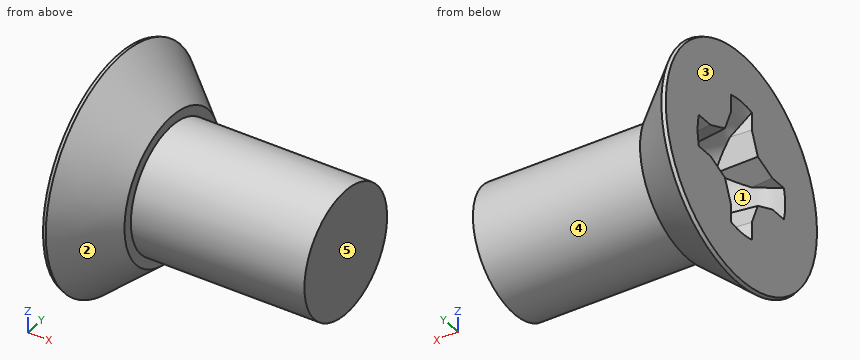
```python
from build123d import *

# Parameters (mm, degrees)
CUT_EXTRUDE1_REACH = 9.904
CIRPATTERN1_COUNT  = 4
DRAFT1_ANGLE       = 5
CHAMFER1_SIZE      = 0.133096
CHAMFER1_SIZE2     = 0.121906137


with BuildPart() as part:
    # Sketch2 → Revolve1 (revolve)
    with BuildSketch(Plane.XY, mode=Mode.PRIVATE) as revolve1_sk:
        Polygon((-3.175, 0), (3.175, 0), (3.175, 1.7526), (-1.6764, 1.7526), (-1.6764, 2.024686895), (-3.175, 3.3274), align=None)
    revolve(revolve1_sk.sketch.rotate(Axis((-3.175, 0, 0), (1, 0, 0)), 180), axis=Axis((-3.175, 0, 0), (1, 0, 0)))

    # Cut-Extrude1: up to this cone (the profile starts inside it)
    cut_extrude1_end = Plane(origin=(-3.175, 0, 0), z_dir=(-1, 0, 0)).offset(-2.137134931) * Cone(1e-06, 12.516790067, 14.398918853, align=(Align.CENTER, Align.CENTER, Align.MIN), mode=Mode.PRIVATE)
    # Sketch3 → Cut-Extrude1 (cut, up to the surface)
    with BuildSketch(Plane.ZY.offset(3.175), mode=Mode.PRIVATE) as cut_extrude1_sk1:
        with BuildLine():
            Line((0, 0), (2.218266667, 0))
            ThreePointArc((2.218266667, 0), (2.207033704, 0.22295568), (2.173448579, 0.443653333))
            Line((2.173448579, 0.443653333), (1.308550956, 0.443653333))
            Line((1.308550956, 0.443653333), (0.696975982, 0.696975982))
            Line((0.696975982, 0.696975982), (0.443653333, 1.308550956))
            Line((0.443653333, 1.308550956), (0.443653333, 2.173448579))
            ThreePointArc((0.443653333, 2.173448579), (0.22295568, 2.207033704), (0, 2.218266667))
            Line((0, 2.218266667), (0, 0))
        make_face()
    cut_extrude1_tool1 = extrude(cut_extrude1_sk1.sketch, amount=-CUT_EXTRUDE1_REACH, mode=Mode.PRIVATE) & cut_extrude1_end
    cut_extrude1 = cut_extrude1_tool1.solids().sort_by_distance((-3.175, 1.109133, 0.031371))[0]
    add(cut_extrude1, mode=Mode.SUBTRACT)

    # CirPattern1: Cut-Extrude1 ×4 about axis
    cirpattern1_axis = Axis((0, 0, 0), (1, 0, 0))
    for i in range(1, CIRPATTERN1_COUNT):
        add(cut_extrude1.rotate(cirpattern1_axis, i * 360 / CIRPATTERN1_COUNT), mode=Mode.SUBTRACT)

    # Draft1
    draft1_faces = [part.faces().sort_by_distance(p)[0] for p in [
        (-2.99204002, 0.443653333, -1.474018435),
        (-2.764573893, 0.582482874, -0.973386795),
        (-2.764573893, 0.973386795, -0.582482874),
        (-2.99204002, 1.474018435, -0.443653333),
        (-2.99204002, 1.474018435, 0.443653333),
        (-2.764573893, 0.973386795, 0.582482874),
        (-2.764573893, 0.582482874, 0.973386795),
        (-2.99204002, 0.443653333, 1.474018435),
        (-2.99204002, -0.443653333, 1.474018435),
        (-2.764573893, -0.582482874, 0.973386795),
        (-2.764573893, -0.973386795, 0.582482874),
        (-2.99204002, -1.474018435, 0.443653333),
        (-2.99204002, -1.474018435, -0.443653333),
        (-2.764573893, -0.973386795, -0.582482874),
        (-2.764573893, -0.582482874, -0.973386795),
        (-2.99204002, -0.443653333, -1.474018435),
    ]]
    draft(draft1_faces, Plane(origin=(-3.175, 0, 0), x_dir=(0, -1, 0), z_dir=(-1, 0, 0)), DRAFT1_ANGLE)

    # Chamfer1
    chamfer1_edges = [part.edges().sort_by_distance(p)[0] for p in [
        (-3.175, 3.3274, 0),
    ]]
    chamfer1_side = [part.faces().sort_by_distance(p)[0] for p in [
        (-2.4257, 2.676043447, 0),
    ]]
    chamfer(chamfer1_edges, length=CHAMFER1_SIZE, length2=CHAMFER1_SIZE2, reference=chamfer1_side[0])


solid = part.part
```
Check sheet for the modelled part. Datum: model origin and axes. Units: mm. Face numbers are marked on the shaded views. A direction names the side the tool comes from. Give positions to 0.01 mm unless a question says otherwise; leave off trailing zeros. Write each loop counter-clockwise with the first axis right and the second up, starting at its lowest first coordinate (ties: lowest second). Pieces come first, ordered by that corner, then holes. Notation, with made-up numbers: (-18.75, 49.25) - (34.25, 49.25) arc R15 cw to (34.25, 63.25) - close; hole circle Ø2 at (48.25, 68.25). An arc over 180 degrees is marked (long way). Answer as a JSON object with one key per item and string values. Group by question number.
1) Access from +Z, -Z, +X, -X, +Y, -Y to the whole of each face (thin tool, end or side, straight path). Record for the marked faces 4 and 5.
2) Thickness scan on probe 1 along X at (y, z) = (0.5, 1.75) (3 decimals); probe 2 along Y at (x, z) = (-2, 1.5); probe 3 along X at (y, z) = (2.75, 1) (3 decimals). Record the ranges inside material, lowest first. Write a range as from..to.
3) Release check for a two-part mould opening along Y. For the marked faces 1, 2 and 3 record: pulls with the +Y half, pulls with the -Y half, needs draft (parallel to the pull), parting line crosses it, or undercut.
4) Sectioned sample at B-B (x = -1.25). Record the cut outline in (y, z).
5) Sectioned sample at A-A (x = -0.25). Record the cut outline in (y, z).
6) Depth check by flat-ended pin: P1, Ø2, axis at x = 2.5, y = -1.5, coming from the +Z side; P2, Ø3, axis at x = 1, y = 0, coming from the +Z side; P3, Ø2, axis at x = 1.5, y = -2, coming from the +Z side. Enter the tip coordinate at first touch or a pass-through.
Geometry results:
{
 "1": {"face 4": "+X", "face 5": "+Z, -Z, +X, +Y, -Y"},
 "2": {"probe 1": "x = -3.175..-1.676", "probe 2": "y = -1.75..1.75", "probe 3": "x = -3.175..-2.713"},
 "3": {"face 1": "undercut", "face 2": "parting line crosses it", "face 3": "needs draft"},
 "4": {"outline": "circle Ø3.51 at (0, 0); hole circle Ø0.37 at (0, 0)"},
 "5": {"outline": "circle Ø3.51 at (0, 0)"},
 "6": {"P1": "stops at z = 1.68", "P2": "stops at z = 1.75", "P3": "stops at z = 1.44"}
}
